For this review, take the finished solid that the model builds, in its own axes (mm). A direction names the side the tool comes from. Coordinates: 2 decimals unless noted, no trailing zeros. Write each loop counter-clockwise with the first axis right and the second up, starting at its lowest first coordinate (ties: lowest second). Pieces come first, ordered by that corner, then holes. Notation, with made-up numbers: (-8.75, 46) -> (-0.75, 46) arc R25 cw to (-0.75, 78) -> close; hole circle Ø3 at (42.25, 66.5). An arc over 180 degrees is marked (long way). Put each result on its own line as item: value. Start each with the question number.
Item 1: For faces 5 (the cylindrical face through (77.267, -3.588, 0.797)), 6 (the flat face through (3, 85, -7.5)), 7 (the flat face through (0, 3, 3)), 8 (the flat face through (3, 85, 0)), 9 (the cylindrical face through (75.133, -12.592, -1.653)), list the 3-axis set-ups (+Z, -Z, +X, -X, +Y, -Y) from which the entire face can be reached by the end or side of a thin tool; tool diameter is ignored.
Item 2: To check wall thickness, follow L1, parallel to Y at x = 105, z = 0 (3 decimals); L2, parallel to Y at x = 52.5, z = 0 (3 decimals); L3, parallel to Y at x = 47.5, z = 2.5. State the ranges of each line that lie inside material, in increasing order.
Item 3: The part is to be moulded in two halves that separate along Y. For faces 1 (the flat face through (-3.758, 78.164, -3.802)), 2 (the flat face through (10.736, 92.658, -3.802)), 3 (the cylindrical face through (60.715, 45.719, 2.753)), 4 (the flat face through (152.4, 3, 3)), say which applies: +Y half, -Y half, draft (parallel to the pull), parting line (faces both ways), or undercut.
Item 4: Consider section B-B on x = 41.5. Give the number of separate pieces and of enclosed holes in the cut face, and give its area (3 significant figures).
Item 5: Insertion check: P1, Ø1.5, axis at x = 17, y = 78, coming from the +Z side; P2, Ø12, axis at y = 21, z = 6, coming from the +X side; P3, Ø10.5, axis at x = 3.5, y = 79.5, coming from the -Z side. Each pin has a flat end and moves straight along its axis. Give the tip position at first contact, or say it passes through.
Item 6: Consider section A-A on x = 123. Give the boundary of the cut face in (y, z) (3 decimals).
```python
from build123d import *

# Parameters (mm, degrees)
SKETCH1_R           = 12.7
BOSS_EXTRUDE1_DEPTH = 152.4
SKETCH7_R           = 12.7
BOSS_EXTRUDE3_DEPTH = 106
SKETCH10_W          = 7.5
SKETCH10_H          = 20.497804761
BOSS_EXTRUDE8_DEPTH = 30
SKETCH11_R          = 3.675
CUT_EXTRUDE2_DEPTH  = 152.4


with BuildPart() as part:
    # Sketch1 → Boss-Extrude1 (new body)
    with BuildSketch(Plane(origin=(0, 0, 0), x_dir=(0, 0, -1), z_dir=(1, 0, 0))):
        with Locations(Location((0, 0, 0), (0, 0, 180))):
            Circle(SKETCH1_R)
    extrude(amount=BOSS_EXTRUDE1_DEPTH)

    # Sketch7 → Boss-Extrude3 (add)
    with BuildSketch(Plane(origin=(44.45, -44.45, 0), x_dir=(0.7071067811865464, 0.7071067811865488, 0), z_dir=(-0.7071067811865488, 0.7071067811865464, 0))):
        with Locations(Location((62.861792847, 0, 0), (0, 0, 90))):
            Circle(SKETCH7_R)
    extrude(amount=BOSS_EXTRUDE3_DEPTH)

    # Sketch10 → Boss-Extrude8 (add)
    with BuildSketch(Plane(origin=(-30.503318806, 30.503318806, 0), x_dir=(0, 0, 1), z_dir=(-0.7071067811865487, 0.7071067811865465, 0))):
        with Locations((-3.75, 62.861792848)):
            Rectangle(SKETCH10_W, SKETCH10_H)
    extrude(amount=BOSS_EXTRUDE8_DEPTH)

    # Sketch11 → Cut-Extrude2 (cut)
    with BuildSketch(Plane(origin=(152.4, 0, 0), x_dir=(0, 0, -1), z_dir=(1, 0, 0))):
        Circle(SKETCH11_R)
    extrude(amount=-CUT_EXTRUDE2_DEPTH, mode=Mode.SUBTRACT)


solid = part.part
```
Return value:
1. face 5: +X, -X
1. face 6: -Z, -X, +Y
1. face 7: +Z, -Z, -X, -Y
1. face 8: +Z, -X, +Y
1. face 9: none
2. L1: -12.7 to -3.675, 3.675 to 12.7
2. L2: -12.7 to -3.675, 3.675 to 12.7, 18.439 to 54.361
2. L3: -12.45 to -2.69, 2.69 to 12.45, 23.79 to 59.01
3. face 1: undercut
3. face 2: +Y half
3. face 3: undercut
3. face 4: draft
4. separate pieces: 2
4. enclosed holes: 1
4. area: 1,180 mm^2
5. P1: z = 12.19
5. P2: x = 90.62
5. P3: z = -7.5
6. outline: circle Ø25.4 at (0, 0); hole circle Ø7.35 at (0, 0)
